Study the drawing (mm; zero at the part's minimum x, y, z) and answer. A direction names the side the tool comes from. Coordinates: 2 decimals unless noted, no trailing zeros. Order: outer loops, then holes, each group sorted by start corner. A loop starts at its lowest first (then second) coordinate and runs counter-clockwise, first axis right, second up. Notation, with made-up numbers: (64.5, 82.5) -> (112.5, 82.5) arc R18 cw to (112.5, 105.5) -> close; hole circle Ø10 at (-2.75, 51). An arc over 180 degrees is marked (long way). Answer in a Markdown table with one row per item. Add a question column.
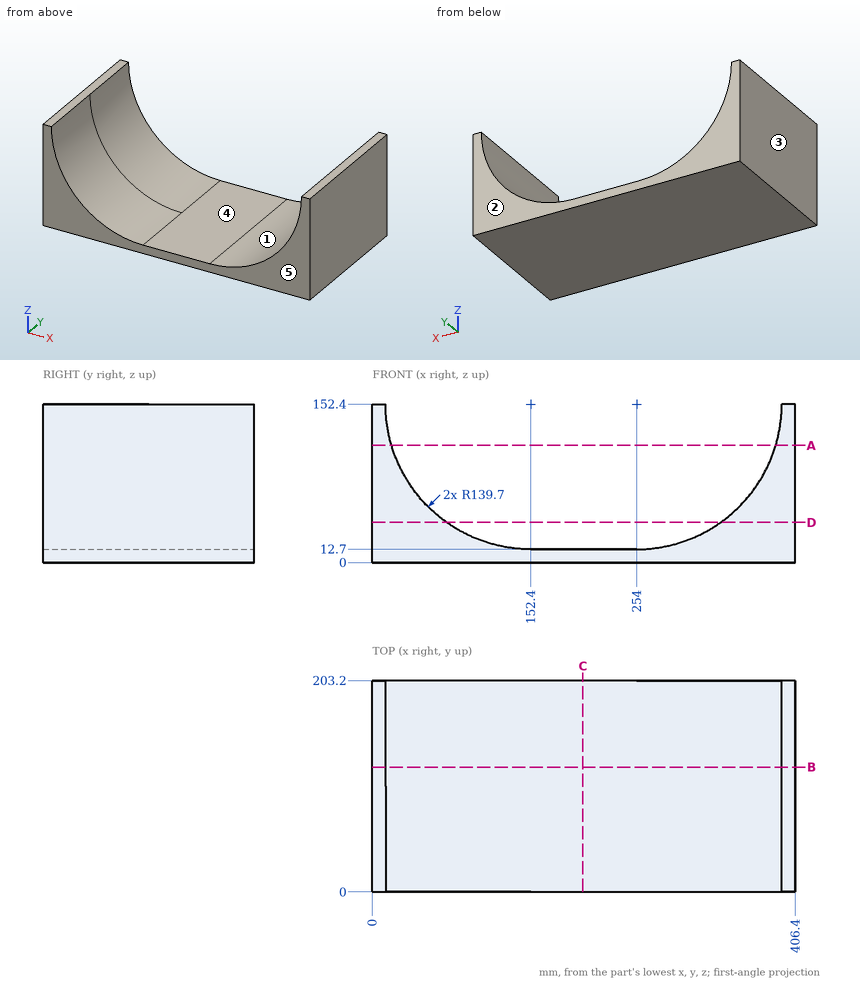
Q1. A cutting plane is placed at D-D (z = 38.5). Determine the outline of the cut face in (x, y), then the cut area to 3 significant figures.
Q2. Determine the mould class of the marked faces 1, 2 and 3 for opening direction X: +X half, -X half, draft (parallel to the pull), parting line (faces both ways), or undercut.
Q3. Given pin 1 (12 mm diameter, centred on x = 138.5, y = 175.5, fed in from +Z); pin 2 (12 mm diameter, centred on x = 109.5, y = 134.5, fed in from +Z), each flat-ended and moving along its own axis, determine where each tip first touches the part or whether it passes through.
Q4. A cutting plane is placed at C-C (x = 202.5). Determine the outline of the cut face in (y, z), then the cut area to 3 significant figures.
Q5. Straight lines are drawn through the part: line 1 (Z direction, x = 232, y = 135.5); line 2 (X direction, y = 38, z = 58.5); line 3 (X direction, y = 30, z = 74). For each, find the intervals that lie inside material, in ascending order.
Q6. For the marked faces 4 and 5, determine the directions among +Z, -Z, +X, -X, +Y, -Y from which every point of the face is accessible in a straight line to the end or side of a thin tool.
Q7. A cutting plane is placed at B-B (y = 120). Determine the outline of the cut face in (x, z), then the cut area to 3 significant figures.
Q8. A cutting plane is placed at A-A (z = 112.5). Determine the outline of the cut face in (x, y).
Returned:
| question | item | result |
|---|---|---|
| 1 | outline | (0, 0) -> (71.51, 0) -> (71.51, 203.2) -> (0, 203.2) -> close; (334.89, 0) -> (406.4, 0) -> (406.4, 203.2) -> (334.89, 203.2) -> close |
| 1 | area | 29,100 mm² |
| 2 | face 1 | undercut |
| 2 | face 2 | draft |
| 2 | face 3 | -X half |
| 3 | pin 1 | stops at z = 14.12 |
| 3 | pin 2 | stops at z = 21.54 |
| 4 | outline | (0, 0) -> (203.2, 0) -> (203.2, 12.7) -> (0, 12.7) -> close |
| 4 | area | 2,580 mm² |
| 5 | line 1 | z = 0 to 12.7 |
| 5 | line 2 | x = 0 to 48.96, 357.44 to 406.4 |
| 5 | line 3 | x = 0 to 36.77, 369.63 to 406.4 |
| 6 | face 4 | +Z, +Y, -Y |
| 6 | face 5 | +Z, -Z, +X, -X, -Y |
| 7 | outline | (0, 0) -> (406.4, 0) -> (406.4, 152.4) -> (393.7, 152.4) arc R139.7 cw to (254, 12.7) -> (152.4, 12.7) arc R139.7 cw to (12.7, 152.4) -> (0, 152.4) -> close |
| 7 | area | 17,100 mm² |
| 8 | outline | (0, 0) -> (18.52, 0) -> (18.52, 203.2) -> (0, 203.2) -> close; (387.88, 0) -> (406.4, 0) -> (406.4, 203.2) -> (387.88, 203.2) -> close |
